```python
from build123d import *

# Parameters (mm, degrees)
ESQUISSE1_R        = 4.5
BOSS_EXTRU_2_DEPTH = 20
ESQUISSE2_R        = 4
BOSS_EXTRU_3_DEPTH = 30
CHANFREIN1_SIZE    = 1


with BuildPart() as part:
    # Esquisse1 → Boss.-Extru.2 (new body)
    with BuildSketch(Plane.XY):
        Circle(ESQUISSE1_R)
    extrude(amount=BOSS_EXTRU_2_DEPTH)

    # Esquisse2 → Boss.-Extru.3 (add)
    with BuildSketch(Plane.XY.offset(20)):
        Circle(ESQUISSE2_R)
    extrude(amount=BOSS_EXTRU_3_DEPTH)

    # Chanfrein1
    chanfrein1_edges = [part.edges().sort_by_distance(p)[0] for p in [
        (-4.5, 0, 0),
        (-4, 0, 50),
    ]]
    chamfer(chanfrein1_edges, length=CHANFREIN1_SIZE)


solid = part.part
```
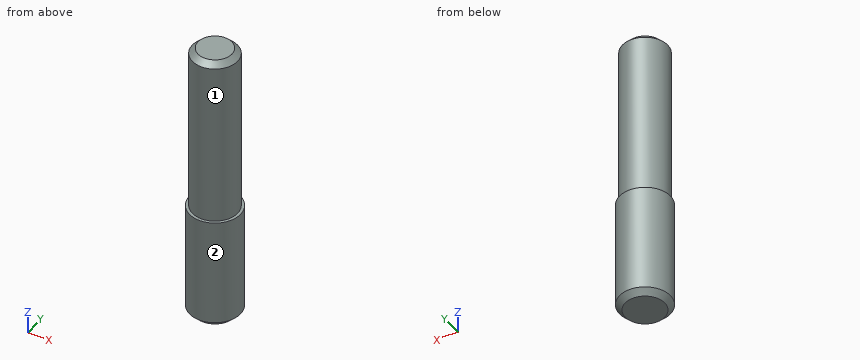
The listing builds one solid part. Answer for the finished solid, in the listing's coordinates (mm). Face numbers are marked on the shaded views. A direction names the side the tool comes from. Round coordinates to 2 decimals unless told otherwise and drop trailing zeros. Order: outer loops, then holes, each group sorted by start corner. A loop starts at its lowest first (then second) coordinate and runs counter-clockwise, first axis right, second up. Notation, with made-up numbers: (-20, 48.25) -> (29, 48.25) arc R22 ccw to (29, 69.25) -> close; hole circle Ø2 at (37, 26.25). An arc over 180 degrees is marked (long way). Answer as CSV lines item,"result".
Q1. A cutting plane is placed at C-C on z = 37. Determine the outline of the cut face in (x, y), plus the area to 3 significant figures.
Computed values:
outline,"circle Ø8 at (0, 0)"
area,"50.3 mm^2"
Q2. Which of the six approach directions +Z, -Z, +X, -X, +Y, -Y give full straight-line access (tool end or side, diameter ignored) to the marked faces 1 and 2?
Computed values:
face 1,"+Z"
face 2,"+Z, -Z"
Q3. Given pin 1 (1.5 mm diameter, centred on y = -3, z = 12.5, fed in from +X); pin 2 (1.5 mm diameter, centred on x = 1.5, z = 41.5, fed in from -Y); pin 3 (4 mm diameter, centred on y = 3, z = 36.5, fed in from -X); pin 4 (1 mm diameter, centred on x = 2, y = -0.5, fed in from -Z), each flat-ended and moving along its own axis, determine where each tip first touches the part or whether it passes through.
Computed values:
pin 1,"stops at x = 3.9"
pin 2,"stops at y = -3.93"
pin 3,"stops at x = -3.87"
pin 4,"stops at z = 0"
Q4. A cutting plane is placed at A-A on y = 0. Determine the outline of the cut face in (x, z).
Computed values:
outline,"(-4.5, 1) -> (-3.5, 0) -> (3.5, 0) -> (4.5, 1) -> (4.5, 20) -> (4, 20) -> (4, 49) -> (3, 50) -> (-3, 50) -> (-4, 49) -> (-4, 20) -> (-4.5, 20) -> close"
Q5. Consider line 1 (Y direction, x = -0.25, z = 39); line 2 (Y direction, x = 1.25, z = 16). Determine where each line is inside the solid, lowest interval first. Write a range as from..to.
Computed values:
line 1,"y = -3.99..3.99"
line 2,"y = -4.32..4.32"
Q6. A cutting plane is placed at D-D on z = 18. Determine the outline of the cut face in (x, y), plus the area to 3 significant figures.
Computed values:
outline,"circle Ø9 at (0, 0)"
area,"63.6 mm^2"
